from build123d import *

# Parameters (mm, degrees)
SKETCH4_R          = 25
CUT_EXTRUDE1_DEPTH = 106
SKETCH5_R          = 3
CUT_EXTRUDE2_DEPTH = 35


with BuildPart() as part:
    # Sketch2 → Revolve2 (revolve)
    with BuildSketch(Plane.XY):
        Polygon((0, 42), (0, -42), (34.886559364, -42), (34.886559364, -32), (32, -32), (32, -20), (30, -20), (30, 20), (32, 20), (32, 32), (34.886559364, 32), (34.886559364, 42), align=None)
    revolve(axis=Axis((0, 42, 0), (0, -1, 0)))

    # Sketch4 → Cut-Extrude1 (cut)
    with BuildSketch(Plane(origin=(0, 42, 0), x_dir=(1, 0, 0), z_dir=(0, 1, 0))):
        Circle(SKETCH4_R)
    extrude(amount=-CUT_EXTRUDE1_DEPTH, mode=Mode.SUBTRACT)

    # Sketch5 → Cut-Extrude2 (cut, symmetric)
    with BuildSketch(Plane(origin=(0, 0, 0), x_dir=(0, 0, -1), z_dir=(1, 0, 0))):
        Circle(SKETCH5_R)
    extrude(amount=CUT_EXTRUDE2_DEPTH, both=True, mode=Mode.SUBTRACT)


solid = part.part
For this review, take the finished solid that the model builds, in its own axes (mm). A direction names the side the tool comes from. Give positions to 0.01 mm unless a question says otherwise; leave off trailing zeros. Write each loop counter-clockwise with the first axis right and the second up, starting at its lowest first coordinate (ties: lowest second). Pieces come first, ordered by that corner, then holes. Notation, with made-up numbers: (87.5, 35) -> (123.5, 35) arc R31 cw to (123.5, 60) -> close; hole circle Ø9 at (76, 64). An arc over 180 degrees is marked (long way). Use CSV: the item, a comma, the result in double quotes.
Q1. Take a section at A-A, the plane x = 0. Write out the cut boundary in (y, z).
Conclusion:
outline,"(-42, -34.89) -> (-32, -34.89) -> (-32, -32) -> (-20, -32) -> (-20, -30) -> (20, -30) -> (20, -32) -> (32, -32) -> (32, -34.89) -> (42, -34.89) -> (42, -25) -> (-42, -25) -> close; (-42, 25) -> (42, 25) -> (42, 34.89) -> (32, 34.89) -> (32, 32) -> (20, 32) -> (20, 30) -> (-20, 30) -> (-20, 32) -> (-32, 32) -> (-32, 34.89) -> (-42, 34.89) -> close"
Q2. To check wall thickness, follow probe 1 along Y at (x, z) = (-27.1, 0); probe 2 along Y at (x, z) = (-28, 16.5); probe 3 along Z at (x, y) = (0, 25). State the ranges of each line that lie inside material, in increasing order. Write a range as [from, to].
Conclusion:
probe 1,"[-42, -3], [3, 42]"
probe 2,"[-42, -32], [32, 42]"
probe 3,"[-32, -25], [25, 32]"
Q3. Take a section at B-B, the plane z = -4.5. Write out the cut boundary in (x, y).
Conclusion:
outline,"(-34.6, -42) -> (-24.59, -42) -> (-24.59, 42) -> (-34.6, 42) -> (-34.6, 32) -> (-31.68, 32) -> (-31.68, 20) -> (-29.66, 20) -> (-29.66, -20) -> (-31.68, -20) -> (-31.68, -32) -> (-34.6, -32) -> close; (24.59, -42) -> (34.6, -42) -> (34.6, -32) -> (31.68, -32) -> (31.68, -20) -> (29.66, -20) -> (29.66, 20) -> (31.68, 20) -> (31.68, 32) -> (34.6, 32) -> (34.6, 42) -> (24.59, 42) -> close"
Q4. Take a section at C-C, the plane y = 0. Write out the cut boundary in (x, z), then the cut area to 3 significant figures.
Conclusion:
outline,"(-29.85, -3) arc R30 ccw to (29.85, -3) -> (24.82, -3) arc R25 cw to (-24.82, -3) -> close; (-29.85, 3) -> (-24.82, 3) arc R25 cw to (24.82, 3) -> (29.85, 3) arc R30 ccw to start"
area,"804 mm2"
Q5. Take a section at D-D, the plane y = 27.5. Write out the cut boundary in (x, z), then the cut area to 3 significant figures.
Conclusion:
outline,"circle Ø64 at (0, 0); hole circle Ø50 at (0, 0)"
area,"1,250 mm2"
Q6. Mouldability with a two-part tool opening along Y and no side actions: class faces 1 (the face through (-27.685, 37.07, -21.228)), 2 (the face through (-9, 20, 29)), 3 (the face through (-15.3, 32, -28.3)), 4 (the face through (8, -42, 24)) as pulls with the +Y half, pulls with the -Y half, needs draft (parallel to the pull), parting line crosses it, or undercut.
Conclusion:
face 1,"needs draft"
face 2,"undercut"
face 3,"undercut"
face 4,"pulls with the -Y half"
Q7. For P1, Ø12, axis at x = 12, z = 16.5, coming from the +Y side; P2, Ø1, axis at x = 15.5, y = 9, coming from the -Z side; P3, Ø1.5, axis at x = -15, y = -22.5, coming from the +Z side; P4, Ø3, axis at y = -22.5, z = -25.5, coming from the -X side, all flat-tipped, find the tip position at first contact; note any pin that passes through.
Conclusion:
P1,"y = 42"
P2,"z = -25.98"
P3,"z = 28.65"
P4,"x = -21.17"
Q8. Tool access review of faces 5 (the face through (27, 0, 3)), 6 (the face through (27.712, 0.28, -11.49)): name each direction out of +Z, -Z, +X, -X, +Y, -Y from which nothing blocks a thin tool from reaching the whole face with its end or side.
Conclusion:
face 5,"+X, -X"
face 6,"none"
